from build123d import *

# Parameters (mm, degrees)
BOSS_EXTRUDE1_DEPTH     = 12.7
SKETCH2_W               = 12.7
SKETCH2_H               = 38.149612403
SKETCH2_W_2             = 38.149612403
SKETCH2_H_2             = 12.7
CUT_EXTRUDE1_DEPTH      = 13.7
SKETCH3_R               = 3.429
CUT_EXTRUDE2_DEPTH      = 13.7
F_1_4_CLEARANCE_HOLE1_D = 6.7564
SKETCH8_W               = 482.6
SKETCH8_H               = 482.6
CUT_EXTRUDE4_DEPTH      = 13.7
SKETCH9_W               = 0.3175
SKETCH9_H               = 38.1
SKETCH9_W_2             = 38.1
SKETCH9_H_2             = 0.3175
CUT_EXTRUDE5_DEPTH      = 13.7


with BuildPart() as part:
    # Sketch1 → Boss-Extrude1 (new body)
    with BuildSketch(Plane(origin=(0, 0, 0), x_dir=(1, 0, 0), z_dir=(0, 1, 0))):
        with BuildLine():
            Line((-406.4, 0), (-482.6, 0))
            ThreePointArc((-482.6, 0), (0, 482.6), (482.6, 0))
            Line((482.6, 0), (406.4, 0))
            ThreePointArc((406.4, 0), (0, 406.4), (-406.4, 0))
        make_face()
    extrude(amount=BOSS_EXTRUDE1_DEPTH)

    # Sketch2 → Cut-Extrude1 (cut, through all)
    with BuildSketch(Plane(origin=(0, 12.7, 0), x_dir=(1, 0, 0), z_dir=(0, 1, 0))):
        with Locations((0, 425.425193799)):
            Rectangle(SKETCH2_W, SKETCH2_H)
        with Locations((425.425193799, 0)):
            Rectangle(SKETCH2_W_2, SKETCH2_H_2)
        with Locations((0, -425.425193799)):
            Rectangle(SKETCH2_W, SKETCH2_H)
        with Locations((-425.425193799, 0)):
            Rectangle(SKETCH2_W_2, SKETCH2_H_2)
    extrude(amount=-CUT_EXTRUDE1_DEPTH, mode=Mode.SUBTRACT)

    # Sketch3 → Cut-Extrude2 (cut, through all)
    with BuildSketch(Plane(origin=(0, 12.7, 0), x_dir=(1, 0, 0), z_dir=(0, 1, 0))):
        with Locations((-6.35, 441.071)):
            Circle(SKETCH3_R)
        with Locations((-441.071, 6.35)):
            Circle(SKETCH3_R)
        with Locations((6.35, 441.071)):
            Circle(SKETCH3_R)
        with Locations((441.071, 6.35)):
            Circle(SKETCH3_R)
    extrude(amount=-CUT_EXTRUDE2_DEPTH, mode=Mode.SUBTRACT)

    # 1/4 Clearance Hole1 (through all)
    with Locations(Plane(origin=(0, 12.7, 0), x_dir=(1, 0, 0), z_dir=(0, 1, 0))):
        with Locations((-365.700877383, 211.1375), (-31.75, 419.1), (-31.75, 450.85), (-419.1, 31.75), (-450.85, 31.75), (-211.1375, 365.700877383)):
            Hole(F_1_4_CLEARANCE_HOLE1_D / 2)

    # Sketch8 → Cut-Extrude4 (cut, through all)
    with BuildSketch(Plane(origin=(0, 12.7, 0), x_dir=(1, 0, 0), z_dir=(0, 1, 0))):
        with Locations((241.3, 241.3)):
            Rectangle(SKETCH8_W, SKETCH8_H)
    extrude(amount=-CUT_EXTRUDE4_DEPTH, mode=Mode.SUBTRACT)

    # Sketch9 → Cut-Extrude5 (cut, through all)
    with BuildSketch(Plane(origin=(0, 12.7, 0), x_dir=(1, 0, 0), z_dir=(0, 1, 0))):
        with Locations((-0.15875, 463.55)):
            Rectangle(SKETCH9_W, SKETCH9_H)
        with Locations((-463.55, 0.15875)):
            Rectangle(SKETCH9_W_2, SKETCH9_H_2)
    extrude(amount=-CUT_EXTRUDE5_DEPTH, mode=Mode.SUBTRACT)


solid = part.part
Design review of the part built by this model. Coordinates are the model's own, in mm. A direction names the side the tool comes from. Coordinates: 2 decimals unless noted, no trailing zeros. Order: outer loops, then holes, each group sorted by start corner. A loop starts at its lowest first (then second) coordinate and runs counter-clockwise, first axis right, second up. Notation, with made-up numbers: (31.5, 11) - (62.5, 11) arc R26 ccw to (62.5, 30) - close; hole circle Ø6 at (37.25, -37.5). An arc over 180 degrees is marked (long way). Put each result on its own line as item: value.
1) Wall thickness on L1, parallel to X at y = 8.25, z = -31.75; L2, parallel to X at y = 5.25, z = -31.5; L3, parallel to Z at x = -180.5, y = 1.5: over which ranges is each line inside the solid? List them lowest first. Write a range as from..to.
Response values:
L1: x = -481.55..-454.23, -447.47..-422.48, -415.72..-405.16
L2: x = -481.57..-454.22, -447.48..-422.47, -415.73..-405.18
L3: z = -447.57..-364.12
2) Take a section at C-C, the plane x = -99.5. Give the boundary of the cut face in (y, z).
Response values:
outline: (0, -472.23) - (12.7, -472.23) - (12.7, -394.03) - (0, -394.03) - close
3) Take a section at A-A, the plane y = 7. Give the boundary of the cut face in (x, z).
Response values:
outline: (-482.6, -0.32) arc R482.6 ccw to (-0.32, -482.6) - (-0.32, -444.5) - (-6.35, -444.5) arc R3.43 cw to (-6.35, -437.64) - (-6.35, -406.35) arc R406.4 cw to (-406.35, -6.35) - (-437.64, -6.35) arc R3.43 cw to (-444.5, -6.35) - (-444.5, -0.32) - close; hole circle Ø6.76 at (-450.85, -31.75); hole circle Ø6.76 at (-419.1, -31.75); hole circle Ø6.76 at (-365.7, -211.14); hole circle Ø6.76 at (-211.14, -365.7); hole circle Ø6.76 at (-31.75, -450.85); hole circle Ø6.76 at (-31.75, -419.1)
4) Tool access review of faces 1 (the face through (-294, 12.7, -296)), 2 (the face through (-422, 6, -6.35)): name each direction out of +Z, -Z, +X, -X, +Y, -Y from which nothing blocks a thin tool from reaching the whole face with its end or side.
Response values:
face 1: +Z, -Z, +X, -X, +Y
face 2: +Z, +X, +Y, -Y
5) Insertion check: P1, Ø6, axis at x = -423, y = 3, coming from the +Z side; P2, Ø4, axis at y = 3, z = -420, coming from the +X side; P3, Ø5, axis at x = -419, y = 3, coming from the -Z side. Each pin has a flat end and moves straight along its axis. Give the tip position at first contact, or say it passes through.
Response values:
P1: stops at z = -6.35
P2: stops at x = -6.35
P3: stops at z = -243.78
6) Take a section at B-B, the plane z = -197. Give the boundary of the cut face in (x, y).
Response values:
outline: (-440.56, 0) - (-355.46, 0) - (-355.46, 12.7) - (-440.56, 12.7) - close
